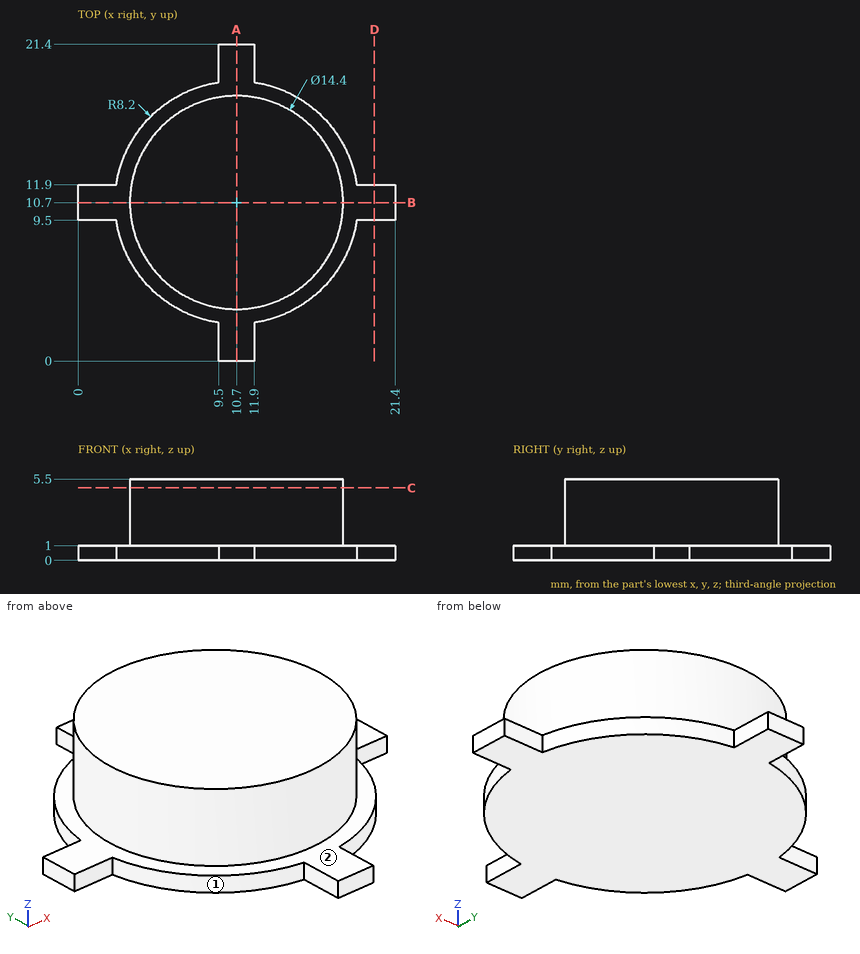
Verification items for this drawing (mm, ordinates from the low corner). A direction names the side the tool comes from. Coordinates: 2 decimals unless noted, no trailing zeros. Loops run counter-clockwise (first coordinate to the right, second up) from the corner with the lowest first, then second, coordinate; pieces in that order, holes last. Notation, with made-up numbers: (-12, 46) - (-4, 46) arc R17 ccw to (-4, 76) - close; hole circle Ø8 at (32.5, -7). An arc over 180 degrees is marked (long way). Answer as a JSON object with one key per item and string values.
(1) Go/stop test with flat-tipped pins: pin 1 Ø0.8 at (x, z) = (19.5, 0.5) entering from -Y; pin 2 Ø1.1 at (x, z) = (19.5, 0.5) entering from +Y; pin 3 Ø1.5 at (x, z) = (13, 4) entering from +Y. Record where each tip stops, or that it passes through.
Response:
{"pin 1": "stops at y = 9.5", "pin 2": "stops at y = 11.9", "pin 3": "stops at y = 17.73"}
(2) Cross-section at C-C, the plane z = 4.9. Record the boundary of the cut face in (x, y), then the cut area to 3 significant figures.
Response:
{"outline": "circle Ø14.4 at (10.7, 10.7)", "area": "163 mm²"}
(3) Cross-section at D-D, the plane x = 20. Record the boundary of the cut face in (y, z).
Response:
{"outline": "(9.5, 0) - (11.9, 0) - (11.9, 1) - (9.5, 1) - close"}
(4) Access from +Z, -Z, +X, -X, +Y, -Y to the whole of each face (thin tool, end or side, straight path). Record for the marked faces 1 and 2.
Response:
{"face 1": "+Z, -Z, -X, -Y", "face 2": "+Z"}
(5) Cross-section at A-A, the plane x = 10.7. Record the boundary of the cut face in (y, z), then the cut area to 3 significant figures.
Response:
{"outline": "(0, 0) - (21.4, 0) - (21.4, 1) - (17.9, 1) - (17.9, 5.5) - (3.5, 5.5) - (3.5, 1) - (0, 1) - close", "area": "86.2 mm²"}
(6) Scan lines: line 1 along Y through (x, z) = (10.75, 3.35); line 2 along Z through (x, y) = (4.25, 6.5); line 3 along X through (y, z) = (13.5, 0.4). Record each from-to range of solid material in increasing order.
Response:
{"line 1": "y = 3.5 to 17.9", "line 2": "z = 0 to 1", "line 3": "x = 2.99 to 18.41"}
